For this review, take the finished solid that the model builds, in its own axes (mm). Face numbers are marked on the shaded views. A direction names the side the tool comes from. Coordinates: 2 decimals unless noted, no trailing zeros. Loops run counter-clockwise (first coordinate to the right, second up) from the corner with the lowest first, then second, coordinate; pieces in that order, holes last. Notation, with made-up numbers: (28, -11) - (67, -11) arc R16 ccw to (67, 19) - close; hole circle Ø11 at (45.5, -32). An arc over 180 degrees is marked (long way). Answer as a JSON object with one key per item and string values. Group by question number.
Item 1: We need section D-D (y = 6). Give the boundary of the cut face in (x, z), then the cut area to 3 significant figures.
Item 2: Clearance check with flat-ended pins moving along their axes: pin 1 (8.5 mm diameter, centred on x = 7, z = 10, fed in from +Y); pin 2 (4 mm diameter, centred on y = 5, z = 10.5, fed in from +X); pin 3 (5 mm diameter, centred on x = 4.42, z = 4, fed in from +Y). State where each tip first meets the part, or that it passes through.
Item 3: We need section C-C (z = 4.75). Give the boundary of the cut face in (x, y).
Item 4: Mouldability with a two-part tool opening along Z and no side actions: class the marked faces 5, 6 and 7 as released by +Z, released by -Z, zero draft, split by the parting line, or undercut.
Item 5: We need section B-B (z = 14). Give the boundary of the cut face in (x, y).
Item 6: Tool access review of the marked faces 1, 2, 3 and 4: name each direction out of +Z, -Z, +X, -X, +Y, -Y from which nothing blocks a thin tool from reaching the whole face with its end or side.
Item 7: To check wall thickness, follow line 1 (X direction, y = 4, z = 11.25); line 2 (Y direction, x = 29, z = 16.75); line 3 (X direction, y = 15.7, z = 14). State the ranges of each line that lie inside material, in increasing order.
Item 8: We need section A-A (x = 8). Give the boundary of the cut face in (y, z), then the cut area to 3 significant figures.
from build123d import *

# Parameters (mm, degrees)
BOSS_EXTRU_1_DEPTH      = 28
ESQUISSE2_R             = 1.6
ENL_V_MAT_EXTRU_1_DEPTH = 53.297323067
ESQUISSE3_R             = 3.05
ENL_V_MAT_EXTRU_2_DEPTH = 54.900371056


with BuildPart() as part:
    # Esquisse1 → Boss.-Extru.1 (new body)
    with BuildSketch(Plane.XY):
        with BuildLine():
            Line((1.5, 0), (18.5, 0))
            ThreePointArc((18.5, 0), (20.267766953, 0.732233047), (21, 2.5))
            Line((21, 2.5), (21, 11.5))
            ThreePointArc((21, 11.5), (21.439339828, 12.560660172), (22.5, 13))
            Line((22.5, 13), (43, 13))
            Line((43, 13), (43, 16.5))
            Line((43, 16.5), (16.079928345, 16.5))
            ThreePointArc((16.079928345, 16.5), (14.645987254, 16.047880111), (13.730696793, 14.855050358))
            Line((13.730696793, 14.855050358), (12.598712706, 11.744949642))
            ThreePointArc((12.598712706, 11.744949642), (11.683422245, 10.552119889), (10.249481154, 10.1))
            Line((10.249481154, 10.1), (2.5, 10.1))
            ThreePointArc((2.5, 10.1), (0.732233047, 9.367766953), (0, 7.6))
            Line((0, 7.6), (0, 7.1))
            Line((0, 7.1), (14, 7.1))
            Line((14, 7.1), (14, 2))
            Line((14, 2), (0, 2))
            Line((0, 2), (0, 1.5))
            ThreePointArc((0, 1.5), (0.439339828, 0.439339828), (1.5, 0))
        make_face()
    extrude(amount=BOSS_EXTRU_1_DEPTH)

    # Esquisse2 → Enlèv. mat.-Extru.1 (cut, through all)
    with BuildSketch(Plane(origin=(0, 10.1, 0), x_dir=(1, 0, 0), z_dir=(0, 1, 0))):
        with Locations(Location((4.42409693, -4, 0), (0, 0, 180))):
            Circle(ESQUISSE2_R)
        with Locations(Location((4.42409693, -24, 0), (0, 0, 180))):
            Circle(ESQUISSE2_R)
    extrude(amount=-ENL_V_MAT_EXTRU_1_DEPTH, mode=Mode.SUBTRACT)

    # Esquisse3 → Enlèv. mat.-Extru.2 (cut, through all)
    with BuildSketch(Plane(origin=(0, 16.5, 0), x_dir=(1, 0, 0), z_dir=(0, 1, 0))):
        with Locations(Location((32.579928345, -14, 0), (0, 0, 270))):
            Circle(ESQUISSE3_R)
        with BuildLine():
            Line((16.079928345, -28), (43, -28))
            Line((43, -28), (43, 0))
            Line((43, 0), (16.079928345, 0))
            Line((16.079928345, 0), (36.818504724, -5.881340534))
            ThreePointArc((36.818504724, -5.881340534), (38.393273299, -6.958588944), (39, -8.767523137))
            Line((39, -8.767523137), (39, -19.232476863))
            ThreePointArc((39, -19.232476863), (38.393273299, -21.041411056), (36.818504724, -22.118659466))
            Line((36.818504724, -22.118659466), (16.079928345, -28))
        make_face()
    extrude(amount=-ENL_V_MAT_EXTRU_2_DEPTH, mode=Mode.SUBTRACT)


solid = part.part
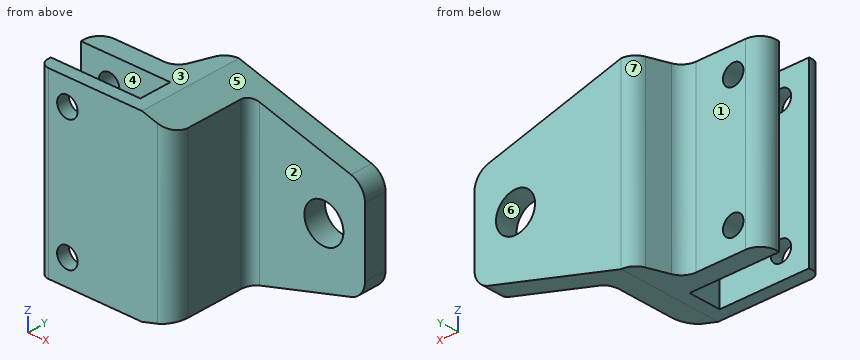
Check sheet entries:
{
 "1": {"outline": "(14, 0) - (16.08, 0) - (21, 1.4) - (21, 26.6) - (16.08, 28) - (14, 28) - close", "area": "189 mm2"},
 "2": {"pin 1": "stops at y = 10.31", "pin 2": "stops at x = 21", "pin 3": "stops at y = 10.1"},
 "3": {"outline": "(0, 1.5) arc R1.5 ccw to (1.5, 0) - (3.01, 0) - (3.01, 2) - (0, 2) - close; (0, 7.1) - (3.01, 7.1) - (3.01, 10.1) - (2.5, 10.1) arc R2.5 ccw to (0, 7.6) - close; (5.84, 0) - (18.5, 0) arc R2.5 ccw to (21, 2.5) - (21, 11.5) arc R1.5 cw to (22.5, 13) - (32.83, 13) - (32.83, 16.5) - (16.08, 16.5) arc R2.5 ccw to (13.73, 14.86) - (12.6, 11.74) arc R2.5 cw to (10.25, 10.1) - (5.84, 10.1) - (5.84, 7.1) - (14, 7.1) - (14, 2) - (5.84, 2) - close"},
 "4": {"face 5": "released by +Z", "face 6": "undercut", "face 7": "zero draft"},
 "5": {"outline": "(0, 1.5) arc R1.5 ccw to (1.5, 0) - (18.5, 0) arc R2.5 ccw to (21, 2.5) - (21, 11.5) arc R1.5 cw to (22.5, 13) - (29.53, 13) - (29.53, 16.5) - (16.08, 16.5) arc R2.5 ccw to (13.73, 14.86) - (12.6, 11.74) arc R2.5 cw to (10.25, 10.1) - (2.5, 10.1) arc R2.5 ccw to (0, 7.6) - (0, 7.1) - (14, 7.1) - (14, 2) - (0, 2) - close; (35.63, 13) - (39, 13) - (39, 16.5) - (35.63, 16.5) - close"},
 "6": {"face 1": "+Z, -Z, -X, +Y", "face 2": "+Z, -Z, +X, -Y", "face 3": "+Z, +X, -X, +Y, -Y", "face 4": "+Z, -Z, -X"},
 "7": {"line 1": "x = 14 to 21", "line 2": "y = 13 to 16.5", "line 3": "x = 14.25 to 29.53, 35.63 to 39"},
 "8": {"outline": "(0, 0) - (2, 0) - (2, 28) - (0, 28) - close; (7.1, 0) - (10.1, 0) - (10.1, 28) - (7.1, 28) - close", "area": "140 mm2"}
}
